from build123d import *

# Parameters (mm, degrees)
SKETCH1_W           = 200
SKETCH1_H           = 300
BOSS_EXTRUDE1_DEPTH = 6.35
SKETCH2_R           = 2.5
SKETCH2_W           = 5
SKETCH2_H           = 15
SKETCH2_W_2         = 15
SKETCH2_H_2         = 5
CUT_EXTRUDE1_DEPTH  = 10
SKETCH3_W           = 5
SKETCH3_H           = 18
CUT_EXTRUDE2_DEPTH  = 10


with BuildPart() as part:
    # Sketch1 → Boss-Extrude1 (new body)
    with BuildSketch(Plane(origin=(0, 0, 0), x_dir=(1, 0, 0), z_dir=(0, 1, 0))):
        with Locations((-100, 150)):
            Rectangle(SKETCH1_W, SKETCH1_H)
        Polygon((-40, 340), (0, 300), (-200, 300), (-160, 340), align=None)
    extrude(amount=BOSS_EXTRUDE1_DEPTH)

    # Sketch2 → Cut-Extrude1 (cut)
    with BuildSketch(Plane.XZ):
        with Locations(Location((-190, -125, 0), (0, 0, 270))):
            Circle(SKETCH2_R)
        with Locations(Location((-130, -10, 0), (0, 0, 270))):
            Circle(SKETCH2_R)
        with Locations(Location((-70, -10, 0), (0, 0, 90))):
            Circle(SKETCH2_R)
        with Locations(Location((-10, -125, 0), (0, 0, 90))):
            Circle(SKETCH2_R)
        with Locations(Location((-70, -290, 0), (0, 0, 270))):
            Circle(SKETCH2_R)
        with Locations(Location((-10, -175, 0), (0, 0, 270))):
            Circle(SKETCH2_R)
        with Locations(Location((-130, -290, 0), (0, 0, 90))):
            Circle(SKETCH2_R)
        with Locations(Location((-190, -175, 0), (0, 0, 90))):
            Circle(SKETCH2_R)
        with Locations((-100, -22.5)):
            Rectangle(SKETCH2_W, SKETCH2_H)
        with Locations((-177.5, -150)):
            Rectangle(SKETCH2_W_2, SKETCH2_H_2)
        with Locations((-22.5, -150)):
            Rectangle(SKETCH2_W_2, SKETCH2_H_2)
    extrude(amount=-CUT_EXTRUDE1_DEPTH, mode=Mode.SUBTRACT)

    # Sketch3 → Cut-Extrude2 (cut)
    with BuildSketch(Plane.XZ):
        with Locations((-177.5, -19)):
            Rectangle(SKETCH3_W, SKETCH3_H)
        with Locations((-177.5, -55)):
            Rectangle(SKETCH3_W, SKETCH3_H)
        with Locations((-177.5, -91)):
            Rectangle(SKETCH3_W, SKETCH3_H)
        with Locations((-22.5, -19)):
            Rectangle(SKETCH3_W, SKETCH3_H)
        with Locations((-22.5, -55)):
            Rectangle(SKETCH3_W, SKETCH3_H)
        with Locations((-22.5, -91)):
            Rectangle(SKETCH3_W, SKETCH3_H)
    extrude(amount=-CUT_EXTRUDE2_DEPTH, mode=Mode.SUBTRACT)


solid = part.part
Design review of the part built by this model. Coordinates are the model's own, in mm. A direction names the side the tool comes from. Round coordinates to 2 decimals unless told otherwise and drop trailing zeros. Write each loop counter-clockwise with the first axis right and the second up, starting at its lowest first coordinate (ties: lowest second). Pieces come first, ordered by that corner, then holes.
Item 1: For faces 1 (the flat face through (-101, 0, -172)), 2 (the flat face through (-175, 3, -19)), list the 3-axis set-ups (+Z, -Z, +X, -X, +Y, -Y) from which the entire face can be reached by the end or side of a thin tool; tool diameter is ignored.
Item 2: Wall thickness on L1, parallel to X at y = 3, z = -175; L2, parallel to Z at x = -130, y = 5.25; L3, parallel to X at y = 4.75, z = -148.5: over which ranges is each line inside the solid? List them lowest first.
Item 3: Draft analysis for pull direction X (two halves, no side actions). For faces 3 (the flat face through (-23, 3, -152.5)), 4 (the flat face through (-200, 3, -148)), 5 (the flat face through (-101, 3, 0)), state which applies: released by +X, released by -X, zero draft, split by the parting line, or undercut.
Item 4: Consider section B-B on y = 3. Count the separate pieces of the cut face and the enclosed holes in it, and give its area (3 significant figures).
Item 5: Consider section A-A on z = -24. Give the boundary of the cut face in (x, y).
Item 6: Consider section C-C on z = -312.5. Give the boundary of the cut face in (x, y).
Item 7: For pin 1 Ø1.5 at (x, y) = (-23, 4.5) entering from -Z; pin 2 Ø6 at (x, z) = (-190, -125) entering from -Y; pin 3 Ø1.5 at (x, y) = (-22, 3.5) entering from -Z, all flat-tipped, find the tip position at first contact; note any pin that passes through.
Item 8: Consider section D-D on x = -166. Give the boundary of the cut face in (y, z).
Check values:
1. face 1: +Z, -Z, +X, -X, -Y
1. face 2: +Y, -Y
2. L1: x = -200 to -192.5, -187.5 to -12.5, -7.5 to 0
2. L2: z = -340 to -292.5, -287.5 to -12.5, -7.5 to 0
2. L3: x = -200 to -185, -170 to -30, -15 to 0
3. face 3: undercut
3. face 4: released by -X
3. face 5: zero draft
4. separate pieces: 1
4. enclosed holes: 17
4. area: 65,500 mm2
5. outline: (-200, 0) - (-180, 0) - (-180, 6.35) - (-200, 6.35) - close; (-175, 0) - (-102.5, 0) - (-102.5, 6.35) - (-175, 6.35) - close; (-97.5, 0) - (-25, 0) - (-25, 6.35) - (-97.5, 6.35) - close; (-20, 0) - (0, 0) - (0, 6.35) - (-20, 6.35) - close
6. outline: (-187.5, 0) - (-12.5, 0) - (-12.5, 6.35) - (-187.5, 6.35) - close
7. pin 1: stops at z = -323.75
7. pin 2: stops at y = 0
7. pin 3: stops at z = -322.75
8. outline: (0, -334) - (6.35, -334) - (6.35, 0) - (0, 0) - close
